Geometry: see drawing. Coordinates: mm, zero at the bounding-box minimum. A direction names the side the tool comes from. Coordinates: 2 decimals unless noted, no trailing zeros. Loops run counter-clockwise (first coordinate to the right, second up) from the corner with the lowest first, then second, coordinate; pieces in that order, holes last. Notation, with made-up numbers: (43, -25) -> (80, -25) arc R20 cw to (80, -6) -> close; hole circle Ø3 at (23.25, 20.5). An arc over 180 degrees is marked (long way). One line per question, with ' | ' between items. Start each with the question number.
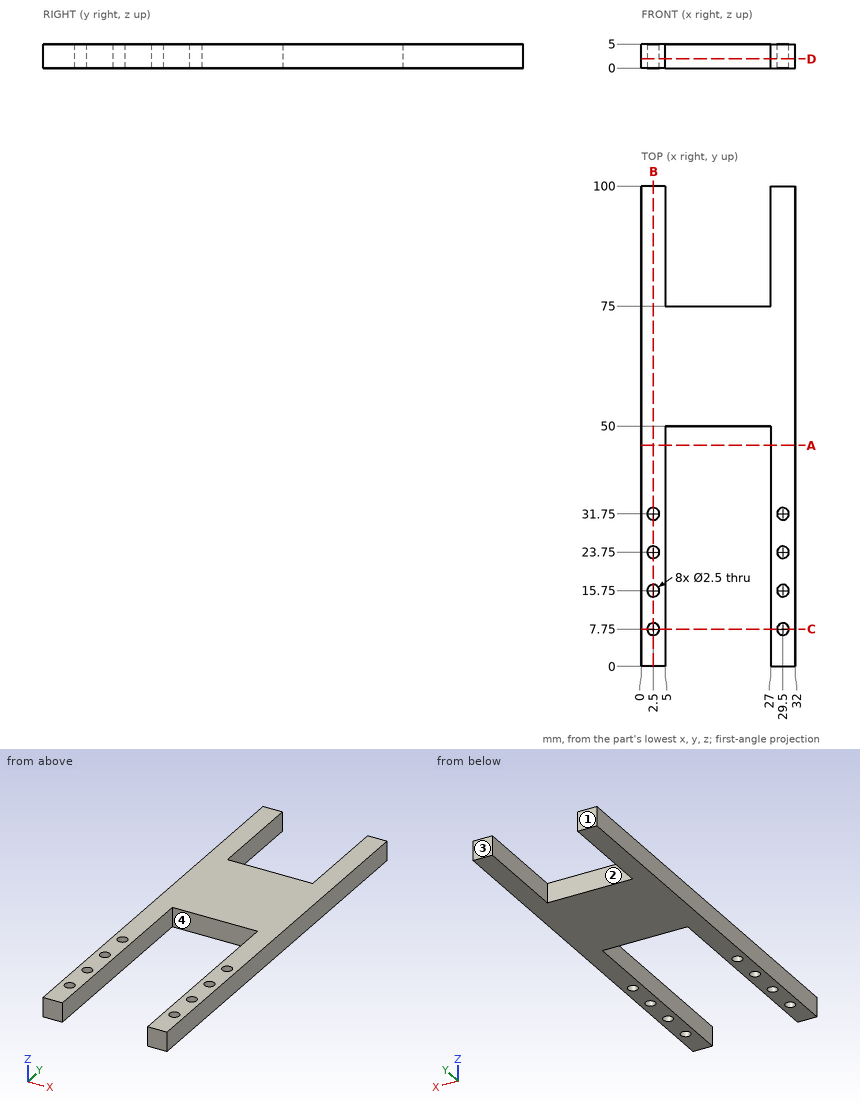
(1) Cut plane D-D, the plane z = 1.9. State how many separate pieces and enclosed holes the cut face has, and give its area (3 significant figures).
(2) Cut plane A-A, the plane y = 46. Return the cut outline in (x, z).
(3) Contact query for flat-ended pins moving along their axis: pin 1 Ø3 at (x, z) = (17.5, 1) entering from +Y; pin 2 Ø2.5 at (x, z) = (14.5, 2.5) entering from -Y. Output: stop coordinate, or through.
(4) Cut plane C-C, the plane y = 7.75. Return the cut outline in (x, z).
(5) Ray query, L1, parallel to Y at x = 2.5, z = 2.8; L2, parallel to X at y = 77, z = 2; L3, parallel to X at y = 8, z = 0.2. Return the intervals inside material, ascending.
(6) Access query for the marked faces 1 and 2. Directions: +Z, -Z, +X, -X, +Y, -Y. A direction counts if a zero-diameter tool reaches every point of the face in a straight line with its end or side. Return the directions, or none.
(7) Draft query along X for the marked faces 3 and 4. Return one class per face: pulls with the +X half, pulls with the -X half, needs draft (parallel to the pull), parting line crosses it, or undercut.
(8) Cut plane B-B, the plane x = 2.5. Return the cut outline in (y, z), and give its area (3 significant figures).
Here are the results:
1) separate pieces: 1 | enclosed holes: 8 | area: 1,510 mm2
2) outline: (0, 0) -> (5, 0) -> (5, 5) -> (0, 5) -> close; (27, 0) -> (32, 0) -> (32, 5) -> (27, 5) -> close
3) pin 1: stops at y = 75 | pin 2: stops at y = 50
4) outline: (0, 0) -> (1.25, 0) -> (1.25, 5) -> (0, 5) -> close; (3.75, 0) -> (5, 0) -> (5, 5) -> (3.75, 5) -> close; (27, 0) -> (28.25, 0) -> (28.25, 5) -> (27, 5) -> close; (30.75, 0) -> (32, 0) -> (32, 5) -> (30.75, 5) -> close
5) L1: y = 0 to 6.5, 9 to 14.5, 17 to 22.5, 25 to 30.5, 33 to 100 | L2: x = 0 to 5, 27 to 32 | L3: x = 0 to 1.28, 3.72 to 5, 27 to 28.28, 30.72 to 32
6) face 1: +Z, -Z, +X, -X, +Y | face 2: +Z, -Z, +Y
7) face 3: needs draft | face 4: undercut
8) outline: (0, 0) -> (6.5, 0) -> (6.5, 5) -> (0, 5) -> close; (9, 0) -> (14.5, 0) -> (14.5, 5) -> (9, 5) -> close; (17, 0) -> (22.5, 0) -> (22.5, 5) -> (17, 5) -> close; (25, 0) -> (30.5, 0) -> (30.5, 5) -> (25, 5) -> close; (33, 0) -> (100, 0) -> (100, 5) -> (33, 5) -> close | area: 450 mm2
